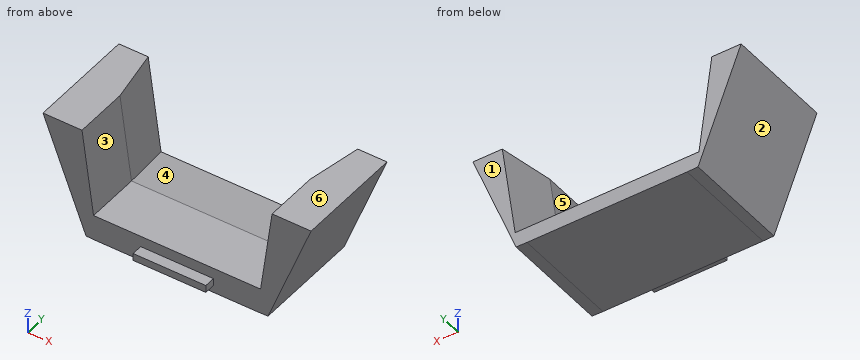
from build123d import *

# Parameters (mm, degrees)
SALIENTE_EXTRUIR1_DEPTH = 30
CORTAR_EXTRUIR2_DEPTH   = 90
CROQUIS5_W              = 20
CROQUIS5_H              = 2
SALIENTE_EXTRUIR2_DEPTH = 3
CHAFL_N1_SIZE           = 15
CHAFL_N1_SIZE2          = 2.644904711
CHAFL_N1_PART_2_SIZE    = 15
CHAFL_N1_PART_2_SIZE2   = 2.644904711
CHAFL_N1_PART_3_SIZE    = 15
CHAFL_N1_PART_3_SIZE2   = 2.644904711


with BuildPart() as part:
    # Croquis2 → Saliente-Extruir1 (new body)
    with BuildSketch(Plane(origin=(0, 0, 0), x_dir=(1, 0, 0), z_dir=(0, 1, 0))):
        Polygon((4.793050572, 35.408576274), (1.793050572, 35.33296049), (-12, 0), (0, 0), (3.845501771, 28.408576274), align=None)
        Polygon((48.793050572, 35.408576274), (4.793050572, 35.408576274), (3.845501771, 28.408576274), (49.740599373, 28.408576274), align=None)
        Polygon((51.793050572, 35.33296049), (48.793050572, 35.408576274), (49.740599373, 28.408576274), (53.586101144, 0), (65.586101144, 0), align=None)
    extrude(amount=SALIENTE_EXTRUIR1_DEPTH)

    # Croquis4 → Cortar-Extruir2 (cut, symmetric)
    with BuildSketch(Plane(origin=(0, 0, 0), x_dir=(0, 0, -1), z_dir=(1, 0, 0))):
        Polygon((0, 0), (5, 0), (5, 30), (-4.90661078, 30), (-4.90661078, 0), align=None)
    extrude(amount=CORTAR_EXTRUIR2_DEPTH, both=True, mode=Mode.SUBTRACT)

    # Croquis5 → Saliente-Extruir2 (add)
    with BuildSketch(Plane(origin=(0, 0, 0), x_dir=(-1, 0, 0), z_dir=(0, -1, 0))):
        with Locations((-26.793050572, 32.408576274)):
            Rectangle(CROQUIS5_W, CROQUIS5_H)
    extrude(amount=SALIENTE_EXTRUIR2_DEPTH)

    # Chaflán1
    chafl_n1_edges = [part.edges().sort_by_distance(p)[0] for p in [
        (26.793050572, 30, -28.408576274),
    ]]
    chafl_n1_side = [part.faces().sort_by_distance(p)[0] for p in [
        (26.793050572, 15, -28.408576274),
    ]]
    chamfer(chafl_n1_edges, length=CHAFL_N1_SIZE, length2=CHAFL_N1_SIZE2, reference=chafl_n1_side[0])

    # Chaflán1 part 2
    chafl_n1_part_2_edges = [part.edges().sort_by_distance(p)[0] for p in [
        (2.261161172, 30, -16.704288137),
    ]]
    chafl_n1_part_2_side = [part.faces().sort_by_distance(p)[0] for p in [
        (2.261161172, 15, -16.704288137),
    ]]
    chamfer(chafl_n1_part_2_edges, length=CHAFL_N1_PART_2_SIZE, length2=CHAFL_N1_PART_2_SIZE2, reference=chafl_n1_part_2_side[0])

    # Chaflán1 part 3
    chafl_n1_part_3_edges = [part.edges().sort_by_distance(p)[0] for p in [
        (51.324939972, 30, -16.704288137),
    ]]
    chafl_n1_part_3_side = [part.faces().sort_by_distance(p)[0] for p in [
        (51.324939972, 15, -16.704288137),
    ]]
    chamfer(chafl_n1_part_3_edges, length=CHAFL_N1_PART_3_SIZE, length2=CHAFL_N1_PART_3_SIZE2, reference=chafl_n1_part_3_side[0])


solid = part.part
Read the model definition and answer for the solid it produces. Units are mm, in the model's axes. Face numbers are marked on the shaded views. A direction names the side the tool comes from. Coordinates: 2 decimals unless noted, no trailing zeros. Loops run counter-clockwise (first coordinate to the right, second up) from the corner with the lowest first, then second, coordinate; pieces in that order, holes last. Notation, with made-up numbers: (71, -32) -> (87, -32) arc R21 ccw to (87, -21) -> close; hole circle Ø7 at (66.5, 71). An arc over 180 degrees is marked (long way). Answer in a Markdown table with one row per item.
Item 1: A cutting plane is placed at B-B on x = 26. Determine the outline of the cut face in (y, z), plus the area to 3 significant figures.
Returned:
| item | result |
|---|---|
| outline | (-3, -33.41) -> (0, -33.41) -> (0, -35.41) -> (30, -35.41) -> (30, -31.05) -> (15, -28.41) -> (0, -28.41) -> (0, -31.41) -> (-3, -31.41) -> close |
| area | 196 mm^2 |
Item 2: For a pull along X with two mould halves and no side action, classify the marked faces 1, 2 and 3 as released by +X, released by -X, zero draft, split by the parting line, or undercut.
Returned:
| item | result |
|---|---|
| face 1 | zero draft |
| face 2 | released by -X |
| face 3 | undercut |
Item 3: For the marked faces 4, 5 and 6, determine the directions among +Z, -Z, +X, -X, +Y, -Y from which every point of the face is accessible in a straight line to the end or side of a thin tool.
Returned:
| item | result |
|---|---|
| face 4 | +Z, +Y |
| face 5 | +Z, +Y, -Y |
| face 6 | +Z, +X, -X, +Y, -Y |
Item 4: A cutting plane is placed at C-C on y = 5. Determine the outline of the cut face in (x, z), plus the area to 3 significant figures.
Returned:
| item | result |
|---|---|
| outline | (-10.05, -5) -> (1.79, -35.33) -> (4.79, -35.41) -> (48.79, -35.41) -> (51.79, -35.33) -> (63.63, -5) -> (52.91, -5) -> (49.74, -28.41) -> (3.85, -28.41) -> (0.68, -5) -> close |
| area | 731 mm^2 |
Item 5: A cutting plane is placed at D-D on z = -26. Determine the outline of the cut face in (x, y).
Returned:
| item | result |
|---|---|
| outline | (-1.85, 0) -> (3.52, 0) -> (3.52, 15) -> (0.85, 30) -> (-1.85, 30) -> close; (50.07, 0) -> (55.44, 0) -> (55.44, 30) -> (52.74, 30) -> (50.07, 15) -> close |
Item 6: A cutting plane is placed at A-A on z = -19. Determine the outline of the cut face in (x, y), plus the area to 3 significant figures.
Returned:
| item | result |
|---|---|
| outline | (-4.58, 0) -> (2.57, 0) -> (2.57, 15) -> (-0.1, 30) -> (-4.58, 30) -> close; (51.01, 0) -> (58.17, 0) -> (58.17, 30) -> (53.68, 30) -> (51.01, 15) -> close |
| area | 389 mm^2 |
Item 7: Straight lines are drawn through the part: line 1 along Z through (x, y) = (45, 11.5); line 2 along Z through (x, y) = (27, -0.5); line 3 along X through (y, z) = (12.5, -18). For each, find the intervals that lie inside material, in ascending order. Write a range as [from, to].
Returned:
| item | result |
|---|---|
| line 1 | z = [-35.41, -28.41] |
| line 2 | z = [-33.41, -31.41] |
| line 3 | x = [-4.97, 2.44], [51.15, 58.56] |
Item 8: Each of these flat-tipped pins is pushed along its axis until it touches: P1, Ø0.9, axis at x = 30.5, y = -1.5, coming from the -Z side; P2, Ø12, axis at x = 26, y = 10.5, coming from the +Z side; P3, Ø1.5, axis at x = 30, y = 19.5, coming from the +Z side. Where does it stop, or does it pass through?
Returned:
| item | result |
|---|---|
| P1 | stops at z = -33.41 |
| P2 | stops at z = -28.41 |
| P3 | stops at z = -29.07 |
